Build history of the part. All positions in model axes, mm. A direction names the side the tool comes from. Round coordinates to 2 decimals unless told otherwise and drop trailing zeros. Write item = value, one per line.
from build123d import *

# Parameters (mm, degrees)
SKETCH_1_R               = 13.75
EXTRUDE_1_DEPTH          = 10
CUT_EXTRUDE_1_DEPTH      = 22.866069606
PATTERN_CIRCULAR_1_COUNT = 20
EXTRUDE_2_DEPTH          = 5
EXTRUDE_2_DEPTH_BACK     = 15
CUT_EXTRUDE_3_DEPTH      = 10
CUT_EXTRUDE_3_DEPTH_BACK = 32
SKETCH_7_W               = 5
SKETCH_7_H               = 34
CUT_EXTRUDE_START        = -22
CUT_EXTRUDE_4_DEPTH      = 22
FILLET_2_R               = 2
FILLET_3_R               = 3
SKETCH_16_R              = 2
CUT_EXTRUDE_5_DEPTH      = 16.5
EXTRUDE_START            = 3.5
SKETCH_18_R              = 5
SKETCH_18_R_2            = 2
EXTRUDE_4_DEPTH          = 3.5
SKETCH_19_R              = 8
CUT_EXTRUDE_7_DEPTH      = 3
FILLET_4_R               = 2
CUT_EXTRUDE_8_DEPTH      = 10
CUT_EXTRUDE_9_DEPTH      = 22
SKETCH_22_R              = 1.5
CUT_EXTRUDE_10_DEPTH     = 22
SKETCH_24_R              = 5
CUT_EXTRUDE_11_DEPTH     = 26
FILLET_5_R               = 10


with BuildPart() as part:
    # 草图1 → 凸台-拉伸1 (new body)
    with BuildSketch(Plane.XY):
        Circle(SKETCH_1_R)
    extrude(amount=EXTRUDE_1_DEPTH)

    # 草图2 → 切除-拉伸1 (cut, through all)
    with BuildSketch(Plane.XY):
        with BuildLine():
            ThreePointArc((0.241645751, 10.934830295), (0, 10.9375), (-0.241645751, 10.934830295))
            add(Edge.make_bspline(
                [(-0.241645751, 10.934830295), (-0.763986756, 11.11684439), (-0.696355124, 11.483892124), (-0.766121321, 11.837511753), (-0.773615233, 11.871945767), (-0.782888612, 11.910793269), (-0.794115121, 11.953996045), (-0.807473925, 12.001489371), (-0.823140069, 12.053203535), (-0.841287339, 12.109063416), (-0.862087187, 12.168988684), (-0.885708875, 12.232893806), (-0.912319248, 12.300688126), (-0.942082628, 12.372275913), (-0.975160664, 12.447556439), (-1.011712206, 12.526424039), (-1.051893167, 12.608768189), (-1.095856396, 12.694473577), (-1.143751548, 12.783420187), (-1.195724957, 12.87548338), (-1.251919512, 12.970533976), (-1.312474533, 13.068438347), (-1.377525652, 13.169058507), (-1.447204695, 13.272252205), (-1.521639564, 13.377873025), (-1.600954126, 13.485770488), (-1.685268101, 13.595790151), (-1.774696952, 13.707773716), (-1.869351783, 13.821559139), (-1.969339231, 13.936980743), (-2.074761371, 14.053869328), (-2.185715611, 14.172052294), (-2.302294605, 14.291353753), (-2.424586158, 14.411594659), (-2.552673133, 14.532592924), (-2.686633373, 14.654163553), (-2.826539612, 14.776118764), (-2.972459398, 14.898268124), (-3.124455015, 15.020418683), (-3.282583418, 15.142375102), (-3.446896124, 15.2639398), (-3.676841988, 15.427049835), (-3.854915516, 15.545415751), (-3.976447477, 15.622814825)],
                knots=[0, 0, 0, 0, 0.165916003, 0.170905922, 0.176663519, 0.183188797, 0.190481754, 0.198542391, 0.207370708, 0.216966704, 0.22733038, 0.238461736, 0.250360771, 0.263027487, 0.276461881, 0.290663956, 0.30563371, 0.321371144, 0.337876258, 0.355149051, 0.373189524, 0.391997677, 0.411573509, 0.431917021, 0.453028213, 0.474907084, 0.497553636, 0.520967867, 0.545149777, 0.570099367, 0.595816637, 0.622301587, 0.649554216, 0.677574526, 0.706362514, 0.735918183, 0.766241531, 0.797332559, 0.829191267, 0.861817654, 0.895211721, 0.929373468, 1, 1, 1, 1], degree=3))
            ThreePointArc((-3.976447477, 15.622814825), (0, 16.120932901), (3.976447477, 15.622814825))
            add(Edge.make_bspline(
                [(0.241645751, 10.934830295), (0.763986756, 11.11684439), (0.696355124, 11.483892124), (0.766121321, 11.837511753), (0.773615233, 11.871945767), (0.782888612, 11.910793269), (0.794115121, 11.953996045), (0.807473925, 12.001489371), (0.823140069, 12.053203535), (0.841287339, 12.109063416), (0.862087187, 12.168988684), (0.885708875, 12.232893806), (0.912319248, 12.300688126), (0.942082628, 12.372275913), (0.975160664, 12.447556439), (1.011712206, 12.526424039), (1.051893167, 12.608768189), (1.095856396, 12.694473577), (1.143751548, 12.783420187), (1.195724957, 12.87548338), (1.251919512, 12.970533976), (1.312474533, 13.068438347), (1.377525652, 13.169058507), (1.447204695, 13.272252205), (1.521639564, 13.377873025), (1.600954126, 13.485770488), (1.685268101, 13.595790151), (1.774696952, 13.707773716), (1.869351783, 13.821559139), (1.969339231, 13.936980743), (2.074761371, 14.053869328), (2.185715611, 14.172052294), (2.302294605, 14.291353753), (2.424586158, 14.411594659), (2.552673133, 14.532592924), (2.686633373, 14.654163553), (2.826539612, 14.776118764), (2.972459398, 14.898268124), (3.124455015, 15.020418683), (3.282583418, 15.142375102), (3.446896124, 15.2639398), (3.676841988, 15.427049835), (3.854915516, 15.545415751), (3.976447477, 15.622814825)],
                knots=[0, 0, 0, 0, 0.165916003, 0.170905922, 0.176663519, 0.183188797, 0.190481754, 0.198542391, 0.207370708, 0.216966704, 0.22733038, 0.238461736, 0.250360771, 0.263027487, 0.276461881, 0.290663956, 0.30563371, 0.321371144, 0.337876258, 0.355149051, 0.373189524, 0.391997677, 0.411573509, 0.431917021, 0.453028213, 0.474907084, 0.497553636, 0.520967867, 0.545149777, 0.570099367, 0.595816637, 0.622301587, 0.649554216, 0.677574526, 0.706362514, 0.735918183, 0.766241531, 0.797332559, 0.829191267, 0.861817654, 0.895211721, 0.929373468, 1, 1, 1, 1], degree=3))
        make_face()
    cut_extrude_1 = extrude(amount=CUT_EXTRUDE_1_DEPTH, mode=Mode.SUBTRACT)

    # 阵列(圆周)1: 切除-拉伸1 ×20 about axis
    pattern_circular_1_axis = Axis((0, 0, -1.5), (0, 0, 1))
    for i in range(1, PATTERN_CIRCULAR_1_COUNT):
        add(cut_extrude_1.rotate(pattern_circular_1_axis, i * 360 / PATTERN_CIRCULAR_1_COUNT), mode=Mode.SUBTRACT)

    # 草图6 → 凸台-拉伸2 (add, two sides: drawn at the far end of the back side and taken through both)
    with BuildSketch(Plane(origin=(0, 0, 0), x_dir=(-1, 0, 0), z_dir=(0, 0, -1)).offset(-EXTRUDE_2_DEPTH_BACK)):
        with BuildLine():
            Line((-4.444597533, -0.703955093), (4.444597533, 0.703955093))
            Line((4.444597533, 0.703955093), (-1.123309149, 35.858334335))
            ThreePointArc((-1.123309149, 35.858334335), (6.18175463, 61.653569146), (-11.311209389, 81.969924763))
            Line((-11.311209389, 81.969924763), (-15.719831619, 70.4850712))
            Line((-15.719831619, 70.4850712), (-10.012504214, 34.45042415))
            Line((-10.012504214, 34.45042415), (-4.444597533, -0.703955093))
        make_face()
    extrude(amount=EXTRUDE_2_DEPTH + EXTRUDE_2_DEPTH_BACK)

    # 草图7 → 切除-拉伸3 (cut, two sides: drawn at the far end of the back side and taken through both)
    with BuildSketch(Plane(origin=(4.444597533, -0.703955093, 0), x_dir=(0, 0, -1), z_dir=(0.9876883405951378, -0.15643446504023126, 0)).offset(-CUT_EXTRUDE_3_DEPTH_BACK)):
        with Locations((2.5, 17)):
            Rectangle(SKETCH_7_W, SKETCH_7_H)
        with Locations((-12.5, 17)):
            Rectangle(SKETCH_7_W, SKETCH_7_H)
    extrude(amount=CUT_EXTRUDE_3_DEPTH + CUT_EXTRUDE_3_DEPTH_BACK, mode=Mode.SUBTRACT)

    # 草图13 → 切除-旋转2 (revolve, cut)
    with BuildSketch(Plane(origin=(12.346104257, -1.955430813, 0), x_dir=(0, 0, 1), z_dir=(-0.9876883405951388, 0.1564344650402244, 0))):
        with BuildLine():
            Line((5, 82.653118449), (5, 34.653118449))
            ThreePointArc((5, 34.653118449), (29, 58.653118449), (5, 82.653118449))
        make_face()
    revolve(axis=Axis((12.41385891, -1.527644771, 5), (0.1564344650402244, 0.9876883405951388, 0)), mode=Mode.SUBTRACT)

    # 草图12 → 切除-拉伸4 (cut)
    with BuildSketch(Plane(origin=(0, 0, -5), x_dir=(-1, 0, 0), z_dir=(0, 0, -1)).offset(CUT_EXTRUDE_START)):
        with BuildLine():
            Line((-11.311209389, 81.969924763), (-11.670273789, 81.03453002))
            ThreePointArc((-11.670273789, 81.03453002), (1.044926137, 71.010674644), (5.846281188, 55.547784376))
            ThreePointArc((5.846281188, 55.547784376), (3.991334875, 45.656412233), (-1.321428913, 37.109213298))
            Line((-1.321428913, 37.109213298), (-1.123309149, 35.858334335))
            ThreePointArc((-1.123309149, 35.858334335), (4.779753161, 44.926816989), (6.848224584, 55.547784376))
            ThreePointArc((6.848224584, 55.547784376), (1.87065393, 71.578181633), (-11.311209389, 81.969924763))
        make_face()
    extrude(amount=CUT_EXTRUDE_4_DEPTH, mode=Mode.SUBTRACT)

    # 圆角2
    fillet_2_edges = [part.edges().sort_by_distance(p)[0] for p in [
        (5.318771811, 33.58140358, 15),
        (5.318771811, 33.58140358, -5),
        (5.318771811, 33.58140358, 0),
        (5.318771811, 33.58140358, 10),
    ]]
    fillet(fillet_2_edges, radius=FILLET_2_R)

    # 圆角3
    fillet_3_edges = [part.edges().sort_by_distance(p)[0] for p in [
        (-5.118751176, 61.808282659, -5),
        (-5.118751176, 61.808282659, 15),
    ]]
    fillet(fillet_3_edges, radius=FILLET_3_R)

    # 草图16 → 切除-拉伸5 (cut)
    with BuildSketch(Plane.XY.offset(10)):
        Circle(SKETCH_16_R)
    extrude(amount=-CUT_EXTRUDE_5_DEPTH, mode=Mode.SUBTRACT)

    # 草图18 → 凸台-拉伸4 (add)
    with BuildSketch(Plane.XY.offset(10).offset(EXTRUDE_START)):
        Circle(SKETCH_18_R)
        Circle(SKETCH_18_R_2, mode=Mode.SUBTRACT)
    extrude(amount=-EXTRUDE_4_DEPTH)

    # 草图19 → 切除-拉伸7 (cut)
    with BuildSketch(Plane(origin=(0, 0, 0), x_dir=(-1, 0, 0), z_dir=(0, 0, -1))):
        Circle(SKETCH_19_R)
    extrude(amount=-CUT_EXTRUDE_7_DEPTH, mode=Mode.SUBTRACT)

    # 圆角4
    fillet_4_edges = [part.edges().sort_by_distance(p)[0] for p in [
        (-5, 0, 10),
    ]]
    fillet(fillet_4_edges, radius=FILLET_4_R)

    # 草图20 → 切除-拉伸8 (cut)
    with BuildSketch(Plane(origin=(0, 0, 0), x_dir=(-1, 0, 0), z_dir=(0, 0, -1))):
        with BuildLine():
            Line((5.774187452, 16.519950341), (3.608867158, 10.324968963))
            ThreePointArc((3.608867158, 10.324968963), (8.919105639, 6.330755157), (10.9375, 0))
            ThreePointArc((10.9375, 0), (10.936832553, -0.120830249), (10.934830295, -0.241645751))
            Line((10.934830295, -0.241645751), (17.498331559, -0.241645751))
            ThreePointArc((17.498331559, -0.241645751), (17.499582885, -0.120825755), (17.5, 0))
            ThreePointArc((17.5, 0), (14.270569022, 10.129208251), (5.774187452, 16.519950341))
        make_face()
    extrude(amount=-CUT_EXTRUDE_8_DEPTH, mode=Mode.SUBTRACT)

    # 草图21 → 切除-拉伸9 (cut)
    with BuildSketch(Plane(origin=(0, 0, 0), x_dir=(-1, 0, 0), z_dir=(0, 0, -1))):
        Polygon((-3.828049486, 14.580673411), (-0.864984465, 15.049976806), (-3.21150144, 29.865301915), (16.542265372, 32.993991216), (24.363988624, -16.390425814), (3.089937746, -19.759904455), (-18.106610022, -23.11710781), (-25.928333274, 26.267309219), (-6.174566462, 29.39599852), align=None)
    extrude(amount=-CUT_EXTRUDE_9_DEPTH, mode=Mode.SUBTRACT)

    # 草图22 → 切除-拉伸10 (cut)
    with BuildSketch(Plane(origin=(1.481532511, -0.234651698, 0), x_dir=(0, 0, -1), z_dir=(0.9876883405951379, -0.15643446504023095, 0))):
        with Locations(Location((-5, 25.5, 0), (0, 0, 90))):
            Circle(SKETCH_22_R)
        with Locations(Location((-5, 19.5, 0), (0, 0, 90))):
            Circle(SKETCH_22_R)
    extrude(amount=-CUT_EXTRUDE_10_DEPTH, mode=Mode.SUBTRACT)

    # 草图24 → 切除-拉伸11 (cut)
    with BuildSketch(Plane(origin=(0, 0, 0), x_dir=(0, 0, 1), z_dir=(-0.9876883405951388, 0.1564344650402244, 0))):
        with Locations(Location((5, 60.060474958, 0), (0, 0, 90))):
            Circle(SKETCH_24_R)
    extrude(amount=CUT_EXTRUDE_11_DEPTH, mode=Mode.SUBTRACT)

    # 圆角5
    # the kernel refuses this fillet: 10 mm, written as the material it takes off along each edge
    with BuildSketch(Plane(origin=(13.61996674, 57.227046138, 5), x_dir=(-0.06465125849803334, -0.4081919812676051, -0.910603932126063), z_dir=(0.1424498389856716, 0.8993928866609987, -0.41328014565975996))) as fillet_5_piece_1:
        with BuildLine():
            CenterArc((28.844410204, 10), FILLET_5_R, 211.965718751, 58.034281249)
            ThreePointArc((20.360760144, 4.705882353), (21.622492356, 2.414788732), (22.627416998, 0))
            Line((22.627416998, 0), (28.844410204, 0))
        make_face()
    revolve(axis=Axis((13.61996674, 57.227046138, 5), (-0.9876883405951378, 0.15643446504023112, 0)), revolution_arc=131.177888663, mode=Mode.SUBTRACT)


solid = part.part
Q1. Cut at A-A, the plane z = 4.25. Give the number of separate pieces and of enclosed holes in the cut face, and give its area (3 significant figures).
Check values:
separate_pieces = 4
enclosed_holes = 0
area = 225 mm²
Q2. Probe probe 1 along Z at (x, y) = (2.75, 68); probe 2 along Y at (x, z) = (3.75, -3); probe 3 along Y at (x, z) = (-3.25, 8.75). List the from-to ranges inside material, lowest first.
Check values:
probe_1 = -5 to -3.89, 13.89 to 15
probe_2 = 33.83 to 41.97, 69.98 to 76.1
probe_3 = 43.93 to 57.98, 64.67 to 67.17
Q3. Mould opens along X. For faces 4 (the face through (7.677, 29.158, 4.93)), 5 (the face through (12.37, 79.21, 5.14)), 6 (the face through (5.27, 34.17, 14.4)) say: released by +X, released by -X, zero draft, split by the parting line, or undercut.
Check values:
face_4 = undercut
face_5 = released by +X
face_6 = released by -X
Q4. Flat gauge pins, fed straight in: pin 1 (5 mm diameter, centred on x = -4, y = 29, fed in from -Z); pin 2 (7 mm diameter, centred on x = 3.5, y = 22.5, fed in from +Z); pin 3 (3 mm diameter, centred on x = -2.5, y = 48, fed in from +Z); pin 4 (10 mm diameter, centred on y = 29, z = 0, fed in from +X). Where does each tip first touch, or does it go through?
Check values:
pin_1 = through
pin_2 = 10
pin_3 = 15
pin_4 = 9.34
Q5. Which spindle directions (+Z, -Z, +X, -X, +Y, -Y) get a long thin tool onto all of the face, cutting with end or side? Do faces 1 (the face through (5.043, 33.625, -2.493)), 2 (the face through (4, 26, 10)), 3 (the face through (1.751, 30.097, 4.93)). Say none if no direction does.
Check values:
face_1 = -Z, -X, -Y
face_2 = +Z, -X, -Y
face_3 = +Z, -Z, -X
